from build123d import *

# Parameters (mm, degrees)
F0_W     = 54
F0_H     = 141
F0_W_2   = 50
F0_H_2   = 137
F1_DEPTH = 33
F2_W     = 54
F2_H     = 2
F3_DEPTH = 141


# Not quite as in the source:
# - the program builds the solid bodies; features that only make, move or delete a surface that nothing else refers to are left out


with BuildPart() as f1:
    # F0 (on Top) → F1 (new body)
    with BuildSketch(Plane.XY):
        with Locations((27, 70.5)):
            Rectangle(F0_W, F0_H)
        with Locations((27, 70.5)):
            Rectangle(F0_W_2, F0_H_2, mode=Mode.SUBTRACT)
    extrude(amount=F1_DEPTH)

    # F2 (on face) → F3 (join)
    with BuildSketch(Plane.XZ):
        with Locations((27, 1)):
            Rectangle(F2_W, F2_H)
    extrude(amount=-F3_DEPTH)


solid = f1.part
Could you check a few things on this model? Use its own coordinates, in mm. A direction names the side the tool comes from. Coordinates: 2 decimals unless noted, no trailing zeros. Order: outer loops, then holes, each group sorted by start corner. A loop starts at its lowest first (then second) coordinate and runs counter-clockwise, first axis right, second up. Notation, with made-up numbers: (-20, 8) -> (13, 8) arc R24 cw to (13, 30) -> close; hole circle Ø3 at (72.25, 84). An arc over 180 degrees is marked (long way). One line per question, with ' | ' between items.
Q1. Imagine slicing it at C-C on y = 26. Please give me the cut outline in (x, z), and give its area (3 significant figures).
Return value:
outline: (0, 0) -> (54, 0) -> (54, 33) -> (52, 33) -> (52, 2) -> (2, 2) -> (2, 33) -> (0, 33) -> close | area: 232 mm²
Q2. If I drill on L1, parallel to Y at x = 39, z = 5.5; L2, parallel to X at y = 56, z = 17; L3, parallel to Z at x = 7, y = 53.5, over which ranges is the centre line in solid material (lowest first)?
Return value:
L1: 0 to 2, 139 to 141 | L2: 0 to 2, 52 to 54 | L3: 0 to 2
Q3. Imagine slicing it at B-B on x = 44. Please give me the cut outline in (y, z), and give its area (3 significant figures).
Return value:
outline: (0, 0) -> (141, 0) -> (141, 33) -> (139, 33) -> (139, 2) -> (2, 2) -> (2, 33) -> (0, 33) -> close | area: 406 mm²
Q4. On a 3-axis mill with a long thin cutter (end or side, diameter ignored), from which of +Z, -Z, +X, -X, +Y, -Y can I reach the whole of each face in a straight line? I mean faces 4 (the face through (52, 70, 17)), 5 (the face through (53, 71, 33)). Say none if no direction works.
Return value:
face 4: +Z | face 5: +Z, +X, -X, +Y, -Y
Q5. Thinking about a two-plate mould opening in X: for faces 1 (the face through (2, 70, 17)), 2 (the face through (27, 141, 16)), 3 (the face through (54, 70, 16)), which applies, pulls with the +X half, pulls with the -X half, needs draft (parallel to the pull), parting line crosses it, or undercut?
Return value:
face 1: undercut | face 2: needs draft | face 3: pulls with the +X half
Q6. Imagine slicing it at A-A on z = 25. Please give me the cut outline in (x, y).
Return value:
outline: (0, 0) -> (54, 0) -> (54, 141) -> (0, 141) -> close; hole (2, 2) -> (52, 2) -> (52, 139) -> (2, 139) -> close
Q7. I'm going to push flat-ended pins straight in: P1, Ø15.5, axis at x = 15.5, z = 17, coming from the -Y side; P2, Ø25, axis at x = 20, y = 58.5, coming from the +Z side. Where does each tip first touch, or does it pass through?
Return value:
P1: y = 0 | P2: z = 2
